from build123d import *

# Parameters (mm, degrees)
F2_R     = 2.7634205328
F2_R_2   = 0.2730680528
F3_DEPTH = 3.175
F4_R     = 0.1905
F5_DEPTH = 1.016
F7_DEPTH = 1.651
F9_DEPTH = 4.5466


# Not quite as in the source:
# - after a boolean that leaves OpenCascade's solid faulty, fix() repairs it


with BuildPart() as f1:
    # F0 (on Front) → F1 (revolve)
    with BuildSketch(Plane.XZ):
        Polygon((0, 3.5306), (0, 0), (9.525, 0), (9.525, 3.048), (8.6543986211, 3.048), (8.4105280196, 3.2918706015), (8.1666574181, 3.048), (7.9227868167, 3.2918706015), (7.6789162152, 3.048), (7.4350456137, 3.2918706015), (7.1911750122, 3.048), (6.9473044108, 3.2918706015), (6.7034338093, 3.048), (6.4595632078, 3.2918706015), (6.2156926063, 3.048), (5.9718220049, 3.2918706015), (5.7279514034, 3.048), (2.1336, 3.048), (1.651, 3.5306), align=None)
    revolve(axis=Axis((4.7625, 0, 0), (1, 0, 0)))

    # F2 (on face) → F3 (cut)
    with BuildSketch(Plane.YZ.offset(9.525)):
        Circle(F2_R)
        Circle(F2_R_2, mode=Mode.SUBTRACT)
    extrude(amount=-F3_DEPTH, mode=Mode.SUBTRACT)

    # F4 (on face) → F5 (join)
    with BuildSketch(Plane(origin=(0, 0, 0), x_dir=(0, -1, 0), z_dir=(-1, 0, 0))):
        Circle(F4_R)
    extrude(amount=F5_DEPTH)

    # F6 (on face) → F7 (join)
    with BuildSketch(Plane(origin=(0, 0, 0), x_dir=(0, -1, 0), z_dir=(-1, 0, 0))):
        with BuildLine():
            ThreePointArc((-2.9561279066, -1.9304), (0, -3.5306), (2.9561279066, -1.9304))
            Line((2.9561279066, -1.9304), (-2.9561279066, -1.9304))
        make_face()
    extrude(amount=F7_DEPTH)

    add(f1.part.fix(), mode=Mode.REPLACE)

    # F8 (on face) → F9 (join)
    with BuildSketch(Plane(origin=(0, 0, 0), x_dir=(0, -1, 0), z_dir=(-1, 0, 0))):
        with BuildLine():
            Line((-1.5521158375, 1.4343592338), (-3.226104454, 1.4343592338))
            ThreePointArc((-3.226104454, 1.4343592338), (-3.4721660307, 0.6396869664), (-3.5254568654, -0.1905))
            Line((-3.5254568654, -0.1905), (-0.6920051213, -0.1905))
            Line((-0.6920051213, -0.1905), (-0.6920051213, 0.3389294034))
            ThreePointArc((-0.6920051213, 0.3389294034), (-1.2486037593, 0.7872849365), (-1.5521158375, 1.4343592338))
        make_face()
        with BuildLine():
            Line((0.6756495639, -0.1905), (3.5254568654, -0.1905))
            ThreePointArc((3.5254568654, -0.1905), (3.4721660307, 0.6396869664), (3.226104454, 1.4343592338))
            Line((3.226104454, 1.4343592338), (1.5521158375, 1.4343592338))
            ThreePointArc((1.5521158375, 1.4343592338), (1.2429873115, 0.7801737537), (0.6756495639, 0.3311225672))
            Line((0.6756495639, 0.3311225672), (0.6756495639, -0.1905))
        make_face()
    extrude(amount=F9_DEPTH)


solid = f1.part
CAD build for the part. Positions are in the model's coordinates, mm. A direction names the side the tool comes from. Coordinates: 2 decimals unless noted, no trailing zeros. Loops run counter-clockwise (first coordinate to the right, second up) from the corner with the lowest first, then second, coordinate; pieces in that order, holes last. Notation, with made-up numbers: (74.5, 43) - (127.5, 43) arc R17 ccw to (127.5, 65) - close; hole circle Ø3 at (-33.75, 32.5). An arc over 180 degrees is marked (long way). Write item = value, one per line. Start each with the question number.
Q1. Which spindle directions (+Z, -Z, +X, -X, +Y, -Y) get a long thin tool onto all of the face, cutting with end or side? Do faces 1 (the flat face through (-1.651, 0, -3)), 2 (the flat face through (6.35, 1, 0)), 3 (the flat face through (-2, -2, -0.19)), 4 (the cylindrical face through (-2.24, -1.25, 0.79)), 5 (the flat face through (-2, 2, 1.434)). Say none if no direction does.
Q2. Flat gauge pins, fed straight in: pin 1 Ø2.5 at (y, z) = (-0.5, 0) entering from -X; pin 2 Ø1.5 at (x, z) = (7.5, 2) entering from -Y; pin 3 Ø0.8 at (x, y) = (-2, -2) entering from +Z; pin 4 Ø0.9 at (x, y) = (-1.5, 2.5) entering from -Z. Where does each tip first touch, or does it go through?
Q3. Cut at A-A, the plane x = 4.25. List the corners of the cut face in (y, z), then the cut area to 3 significant figures.
Q4. Drill centre lines: L1, parallel to X at y = -1.75, z = -1; L2, parallel to X at y = 2, z = 0.5; L3, parallel to Y at x = 6, z = -0.5. Where is each one in solid material? Low to high.
Q5. Cut at B-B, the plane x = 1. List the corners of the cut face in (y, z).
Q6. Pull direction Y, two halves, no side cores. Call faces 6 (the cylindrical face through (-2.241, 1.242, 0.779)), 7 (the cylindrical face through (9.08, -3.02, -0.4)), 8 (the flat face through (-2, 2, -0.19)): pulls with the +Y half, pulls with the -Y half, needs draft (parallel to the pull), parting line crosses it, or undercut.
Computed:
q1.face_1 = -Z, -X, +Y, -Y
q1.face_2 = +X
q1.face_3 = -X, +Y, -Y
q1.face_4 = +Z, -X
q1.face_5 = +Z, -X, +Y, -Y
q2.pin_1 = -4.55
q2.pin_2 = -3.04
q2.pin_3 = 1.43
q2.pin_4 = -2.87
q3.outline = circle Ø6.1 at (0, 0)
q3.area = 29.2 mm²
q4.L1 = 0 to 6.35
q4.L2 = -4.55 to 6.35
q4.L3 = -3.23 to 3.23
q5.outline = circle Ø7.06 at (0, 0)
q6.face_6 = undercut
q6.face_7 = parting line crosses it
q6.face_8 = needs draft
